Source: CAD feature listing. Evaluate the final solid. Frame: model axes, mm. A direction names the side the tool comes from. Round coordinates to 2 decimals unless told otherwise and drop trailing zeros. Order: outer loops, then holes, each group sorted by start corner. A loop starts at its lowest first (then second) coordinate and runs counter-clockwise, first axis right, second up. Notation, with made-up numbers: (64, 69.5) - (100, 69.5) arc R30 ccw to (100, 100.5) - close; hole circle Ø5 at (19.25, 23). An arc over 180 degrees is marked (long way). Use one line per item in the form item = value. Start each with the question number.
Q1. Cut plane D-D, the plane x = -25. Return the cut outline in (y, z) (3 decimals), and give its area (4 significant figures).
Q2. Set-up query: faces 1 (the flat face through (22, 7, 1)), 2 (the flat face through (-25, -8.25, 2)), 3 (the flat face through (26, 0, 2)). Return all of +Z, -Z, +X, -X, +Y, -Y with unobstructed straight access to the full face (end or side cutting, diameter ignored); none if empty.
Q3. Cut plane B-B, the plane x = 31. Return the cut outline in (y, z) (3 decimals), and give its area (3 significant figures).
Q4. Draft query along Y for faces 4 (the flat face through (38, 11, 1)), 5 (the flat face through (-2, 0, 2)), 6 (the flat face through (-23, -9, 2)). Return one class per face: released by +Y, released by -Y, zero draft, split by the parting line, or undercut.
Q5. Cut plane C-C, the plane z = 0.6. Give the number of separate pieces and of enclosed holes in the cut face, and give its area (3 significant figures).
Q6. Ray query, line 1 (X direction, y = 7.5, z = 0.3); line 2 (Y direction, x = -22.5, z = 1.15); line 3 (Y direction, x = 31, z = 1.5) (3 decimals). Return the intervals inside material, ascending. Write a range as [from, to].
Q7. Cut plane A-A, the plane y = 0. Return the cut outline in (x, z) (3 decimals).
Q8. Pin query (flat end, axial travel): pin 1 Ø2.5 at (x, y) = (38, 7) entering from +Z; pin 2 Ø1.6 at (y, z) = (-11.5, 1) entering from +X; pin 3 Ø1 at (y, z) = (9, 2) entering from +X; pin 4 Ø1 at (y, z) = (-0.5, 2) entering from -X. Return the tip coordinate at first contact, or that it passes through.
from build123d import *

# Parameters (mm, degrees)
SKETCH1_R           = 1.625
SKETCH1_R_2         = 3.5
SKETCH1_R_3         = 1.125
SKETCH1_W           = 8
SKETCH1_H           = 4
BOSS_EXTRUDE1_DEPTH = 2
SKETCH8_R           = 1.125
BOSS_EXTRUDE4_DEPTH = 1.5


with BuildPart() as part:
    # Sketch1 → Boss-Extrude1 (new body)
    with BuildSketch(Plane.XY):
        with BuildLine():
            Line((-27, -8.25), (-27, -12.25))
            Line((-27, -12.25), (38, -12.25))
            Line((38, -12.25), (38, -10))
            ThreePointArc((38, -10), (48, 0), (38, 10))
            Line((38, 10), (38, 12.25))
            Line((38, 12.25), (-27, 12.25))
            Line((-27, 12.25), (-27, 8.25))
            Line((-27, 8.25), (-23, 8.25))
            Line((-23, 8.25), (-23, 10.25))
            Line((-23, 10.25), (-4.001411983, 10.429151381))
            Line((-4.001411983, 10.429151381), (-2, 10.429151381))
            Line((-2, 10.429151381), (-2, -10.070848619))
            Line((-2, -10.070848619), (-4.001411983, -10.070848619))
            Line((-4.001411983, -10.070848619), (-23, -10.25))
            Line((-23, -10.25), (-23, -8.25))
            Line((-23, -8.25), (-27, -8.25))
        make_face()
        with Locations((38, 7)):
            Circle(SKETCH1_R, mode=Mode.SUBTRACT)
        with Locations((45, 0)):
            Circle(SKETCH1_R, mode=Mode.SUBTRACT)
        with Locations((38, -7)):
            Circle(SKETCH1_R, mode=Mode.SUBTRACT)
        with Locations((31, 0)):
            Circle(SKETCH1_R, mode=Mode.SUBTRACT)
        with Locations((38, 0)):
            Circle(SKETCH1_R_2, mode=Mode.SUBTRACT)
        with Locations((-25, 10.25)):
            Circle(SKETCH1_R_3, mode=Mode.SUBTRACT)
        with Locations((-25, -10.25)):
            Circle(SKETCH1_R_3, mode=Mode.SUBTRACT)
        with Locations((0, 10.429151381)):
            Circle(SKETCH1_R_3, mode=Mode.SUBTRACT)
        with Locations((0, -10.070848619)):
            Circle(SKETCH1_R_3, mode=Mode.SUBTRACT)
        with Locations((18, 7)):
            Rectangle(SKETCH1_W, SKETCH1_H, mode=Mode.SUBTRACT)
        with Locations((18, -7)):
            Rectangle(SKETCH1_W, SKETCH1_H, mode=Mode.SUBTRACT)
    extrude(amount=BOSS_EXTRUDE1_DEPTH)

    # Sketch8 → Boss-Extrude4 (add)
    with BuildSketch(Plane.XY.offset(2)):
        Polygon((-27, 12.25), (5.5, 12.25), (5.5, -12.25), (-27, -12.25), (-27, -8.25), (-23, -8.25), (-23, -10.25), (-2, -10.070848619), (-2, 10.429151381), (-23, 10.25), (-23, 8.25), (-27, 8.25), align=None)
        with Locations((-25, 10.25)):
            Circle(SKETCH8_R, mode=Mode.SUBTRACT)
        with Locations((-25, -10.25)):
            Circle(SKETCH8_R, mode=Mode.SUBTRACT)
        with Locations((0, 10.429151381)):
            Circle(SKETCH8_R, mode=Mode.SUBTRACT)
        with Locations((0, -10.070848619)):
            Circle(SKETCH8_R, mode=Mode.SUBTRACT)
    extrude(amount=BOSS_EXTRUDE4_DEPTH)


solid = part.part
Completed:
q1.outline = (-12.25, 0) - (-11.375, 0) - (-11.375, 3.5) - (-12.25, 3.5) - close; (-9.125, 0) - (-8.25, 0) - (-8.25, 3.5) - (-9.125, 3.5) - close; (8.25, 0) - (9.125, 0) - (9.125, 3.5) - (8.25, 3.5) - close; (11.375, 0) - (12.25, 0) - (12.25, 3.5) - (11.375, 3.5) - close
q1.area = 12.25 mm2
q2.face_1 = +Z, -Z
q2.face_2 = +Z, -Z, -X
q2.face_3 = +Z, +X, +Y, -Y
q3.outline = (-12.25, 0) - (-1.625, 0) - (-1.625, 2) - (-12.25, 2) - close; (1.625, 0) - (12.25, 0) - (12.25, 2) - (1.625, 2) - close
q3.area = 42.5 mm2
q4.face_4 = zero draft
q4.face_5 = undercut
q4.face_6 = undercut
q5.separate_pieces = 1
q5.enclosed_holes = 11
q5.area = 1,100 mm2
q6.line_1 = [-2, 14], [22, 36.45], [39.55, 44.61]
q6.line_2 = [-12.25, -10.25], [10.25, 12.25]
q6.line_3 = [-12.25, -1.625], [1.625, 12.25]
q7.outline = (-2, 0) - (29.375, 0) - (29.375, 2) - (5.5, 2) - (5.5, 3.5) - (-2, 3.5) - close; (32.625, 0) - (34.5, 0) - (34.5, 2) - (32.625, 2) - close; (41.5, 0) - (43.375, 0) - (43.375, 2) - (41.5, 2) - close; (46.625, 0) - (48, 0) - (48, 2) - (46.625, 2) - close
q8.pin_1 = through
q8.pin_2 = 38
q8.pin_3 = 43.27
q8.pin_4 = -2
